Design review of the part shown in the three views and the two pictorial views. Dimensions are in mm from the part's minimum x, y and z. Coordinates: 2 decimals unless noted, no trailing zeros. Write each loop counter-clockwise with the first axis right and the second up, starting at its lowest first coordinate (ties: lowest second). Pieces come first, ordered by that corner, then holes. Notation, with made-up numbers: (17.5, 50.5) - (22.5, 50.5) arc R13 ccw to (22.5, 74.5) - close; hole circle Ø8 at (-28.5, 35). An arc over 180 degrees is marked (long way). Return JSON: item names as keys, results as strings. Group by question number.
(1) We need section C-C on z = 2.9. State the section outline as (x, y) points.
(2) To check wall thickness, follow L1, parallel to X at y = 24.5, z = 2.6; L2, parallel to Y at x = 51, z = 2.85. State the ranges of each line that lie inside material, in increasing order. Write a range as from..to.
(3) For pin 1 Ø0.6 at (y, z) = (35, 3) entering from -X; pin 2 Ø1 at (x, z) = (19.5, 3) entering from -Y; pin 3 Ø1 at (x, z) = (34.5, 3) entering from +Y, all flat-tipped, find the tip position at first contact; note any pin that passes through.
(4) We need section A-A on y = 7. State the section outline as (x, z) points.
(5) We need section B-B on x = 50. State the section outline as (y, z) points, then the cut area to 3 significant figures.
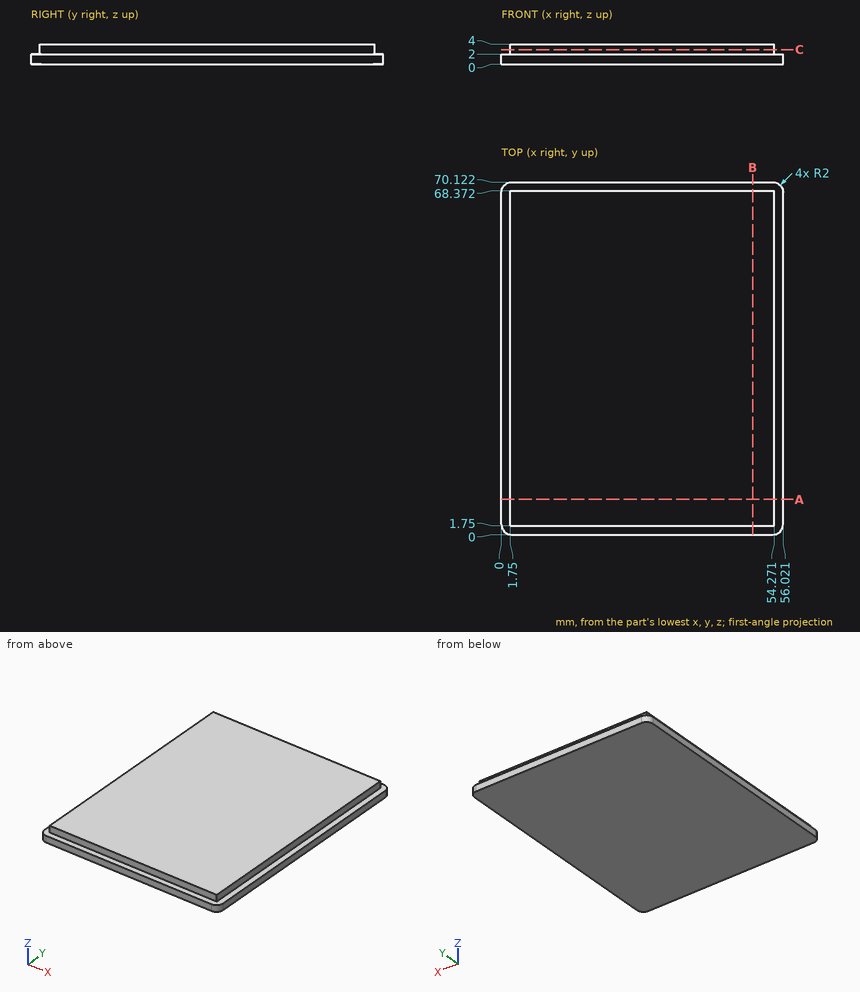
Ans:
{
 "1": {"outline": "(1.75, 1.75) - (54.27, 1.75) - (54.27, 68.37) - (1.75, 68.37) - close"},
 "2": {"L1": "1.75..54.27", "L2": "1.75..68.37"},
 "3": {"pin 1": "x = 1.75", "pin 2": "y = 1.75", "pin 3": "y = 68.37"},
 "4": {"outline": "(0, 0) - (56.02, 0) - (56.02, 2) - (54.27, 2) - (54.27, 4) - (1.75, 4) - (1.75, 2) - (0, 2) - close"},
 "5": {"outline": "(0, 0) - (70.12, 0) - (70.12, 2) - (68.37, 2) - (68.37, 4) - (1.75, 4) - (1.75, 2) - (0, 2) - close", "area": "273 mm²"}
}
